Source: CAD feature listing. Evaluate the final solid. Frame: model axes, mm. Face numbers are marked on the shaded views. A direction names the side the tool comes from. Give positions to 0.01 mm unless a question says otherwise; leave off trailing zeros. Loops run counter-clockwise (first coordinate to the right, second up) from the corner with the lowest first, then second, coordinate; pieces in that order, holes last.
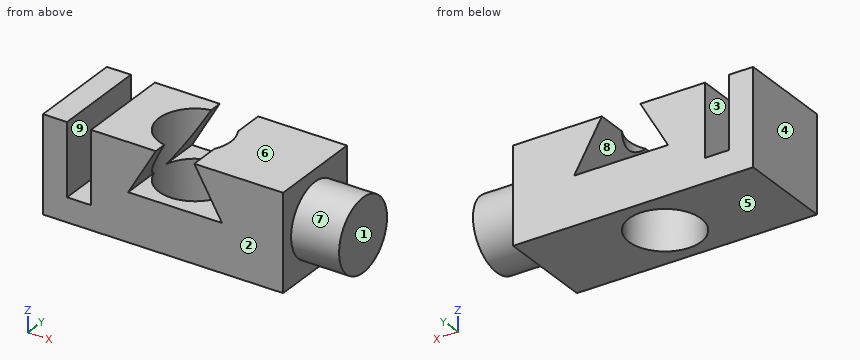
```python
from build123d import *

# Parameters (mm, degrees)
F0_W     = 50
F0_H     = 20
F0_R     = 7.5
F1_DEPTH = 20
F2_W     = 5
F2_H     = 20
F3_DEPTH = 15
F5_DEPTH = 20.001
F6_R     = 7.5
F7_DEPTH = 10


with BuildPart() as f1:
    # F0 (on Top) → F1 (new body)
    with BuildSketch(Plane.XY):
        Rectangle(F0_W, F0_H)
        Circle(F0_R, mode=Mode.SUBTRACT)
    extrude(amount=F1_DEPTH)

    # F2 (on face) → F3 (cut)
    with BuildSketch(Plane.XY.offset(20)):
        with Locations((-17.5, 0)):
            Rectangle(F2_W, F2_H)
    extrude(amount=-F3_DEPTH, mode=Mode.SUBTRACT)

    # F4 (on face) → F5 (cut, through all)
    with BuildSketch(Plane.XZ.offset(10)):
        Polygon((6.5, 20), (-1.5, 20), (-7.273503, 10), (12.273503, 10), align=None)
    extrude(amount=-F5_DEPTH, mode=Mode.SUBTRACT)

    # F6 (on face) → F7 (join)
    with BuildSketch(Plane.YZ.offset(25)):
        with Locations((0, 10)):
            Circle(F6_R)
    extrude(amount=F7_DEPTH)


solid = f1.part
```
(1) Section C-C, the plane z = 13.75. Return the cut outline in (x, y).
A:
outline: (-25, -10) - (-20, -10) - (-20, 10) - (-25, 10) - close; (-15, -10) - (-5.11, -10) - (-5.11, -5.49) arc R7.5 cw to (-5.11, 5.49) - (-5.11, 10) - (-15, 10) - close; (10.11, -10) - (25, -10) - (25, -6.5) - (35, -6.5) - (35, 6.5) - (25, 6.5) - (25, 10) - (10.11, 10) - close
(2) Mould query, pull axis X, two halves, no side actions, for the marked faces 1, 2, 3 and 4. Classes: pulls with the +X half, pulls with the -X half, needs draft (parallel to the pull), parting line crosses it, or undercut.
A:
face 1: pulls with the +X half
face 2: needs draft
face 3: undercut
face 4: pulls with the -X half
(3) Ray query, line 1 along Y through (x, z) = (0, 5.5); line 2 along X through (y, z) = (5.5, 17); line 3 along X through (y, z) = (3, 16.75). Return the intervals inside material, ascending.
A:
line 1: y = -10 to -7.5, 7.5 to 10
line 2: x = -25 to -20, -15 to -5.1, 8.23 to 25
line 3: x = -25 to -20, -15 to -6.87, 8.38 to 35
(4) Section D-D, the plane y = -8.25. Return the cut outline in (x, z), then the cut area to 3 significant figures.
A:
outline: (-25, 0) - (25, 0) - (25, 20) - (6.5, 20) - (12.27, 10) - (-7.27, 10) - (-1.5, 20) - (-15, 20) - (-15, 5) - (-20, 5) - (-20, 20) - (-25, 20) - close
area: 787 mm2
(5) Section B-B, the plane y = 0. Return the cut outline in (x, z), then the cut area to 3 significant figures.
A:
outline: (-25, 0) - (-7.5, 0) - (-7.5, 20) - (-15, 20) - (-15, 5) - (-20, 5) - (-20, 20) - (-25, 20) - close; (7.5, 0) - (25, 0) - (25, 2.5) - (35, 2.5) - (35, 17.5) - (25, 17.5) - (25, 20) - (7.5, 20) - (7.5, 18.27) - (12.27, 10) - (7.5, 10) - close
area: 755 mm2
(6) Reachability of the marked faces 5, 6, 7, 8 and 9 from +Z, -Z, +X, -X, +Y, -Y: full face, straight path, thin tool, end or side. Return the list, or none.
A:
face 5: -Z, +X, -X, +Y, -Y
face 6: +Z, +X, -X, +Y, -Y
face 7: +X
face 8: +Y, -Y
face 9: +Z, +Y, -Y
(7) Section A-A, the plane x = 0. Return the cut outline in (y, z), then the cut area to 3 significant figures.
A:
outline: (-10, 0) - (-7.5, 0) - (-7.5, 10) - (-10, 10) - close; (7.5, 0) - (10, 0) - (10, 10) - (7.5, 10) - close
area: 50.0 mm2
